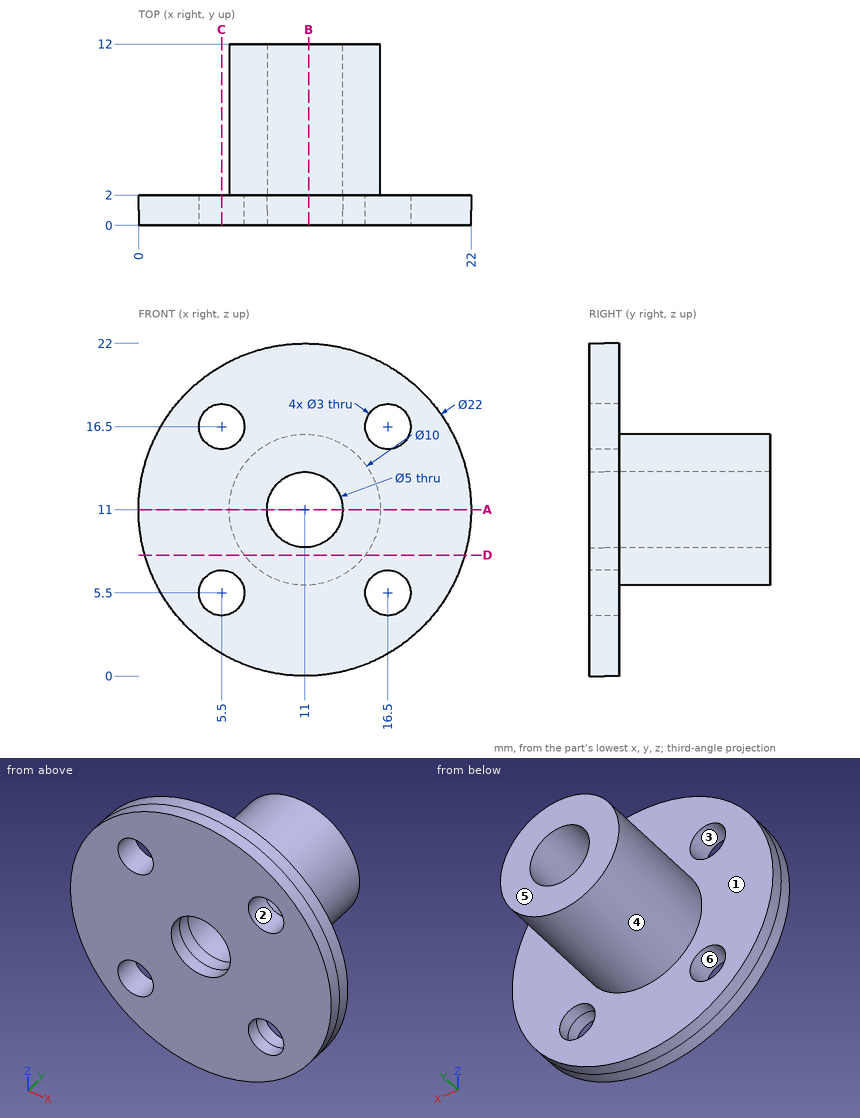
Part print with two shaded views. Sizes in mm from the minimum x, y, z corner. A direction names the side the tool comes from. Coordinates: 2 decimals unless noted, no trailing zeros. Write each loop counter-clockwise with the first axis right and the second up, starting at its lowest first coordinate (ties: lowest second). Pieces come first, ordered by that corner, then holes. Notation, with made-up numbers: (38, -8.75) -> (47, -8.75) arc R12 ccw to (47, 4.25) -> close; hole circle Ø10 at (-17, 51.5). An arc over 180 degrees is marked (long way). Return JSON: item names as keys, results as strings. Group by question number.
Q1. Flat gauge pins, fed straight in: pin 1 (2.5 mm diameter, centred on x = 16.5, z = 5.5, fed in from -Y); pin 2 (3 mm diameter, centred on y = 4, z = 7.5, fed in from -X); pin 3 (1.5 mm diameter, centred on y = 8.5, z = 11.5, fed in from -X); pin 4 (3.5 mm diameter, centred on x = 5.5, z = 5.5, fed in from +Y). Where does each tip first touch, or does it go through?
Q2. Drill centre lines: line 1 (X direction, y = 5.5, z = 11); line 2 (Z direction, x = 11, y = 0.5); line 3 (Y direction, x = 13, z = 2.25). Where is each one in solid material? Low to high.
Q3. Cut at B-B, the plane x = 11.25. Give the cut face in (y, z).
Q4. Cut at A-A, the plane z = 11. Give the cut face in (x, y), then the cut area to 3 significant figures.
Q5. Which spindle directions (+Z, -Z, +X, -X, +Y, -Y) get a long thin tool onto all of the face, cutting with end or side? Do the marked faces 1 and 2. Say none if no direction does.
Q6. Cut at D-D, the plane z = 8. Give the cut face in (x, y).
Q7. Pull direction Z, two halves, no side cores. Call the marked faces 3, 4, 5 and 6: released by +Z, released by -Z, zero draft, split by the parting line, or undercut.
Q8. Cut at C-C, the plane x = 5.5. Give the cut face in (y, z).
Returned:
{
 "1": {"pin 1": "passes through", "pin 2": "stops at x = 6.42", "pin 3": "stops at x = 6", "pin 4": "stops at y = 2"},
 "2": {"line 1": "x = 6 to 8.5, 13.5 to 16", "line 2": "z = 0 to 8.5, 13.5 to 22", "line 3": "y = 0 to 2"},
 "3": {"outline": "(0, 0) -> (2, 0) -> (2, 6.01) -> (12, 6.01) -> (12, 8.51) -> (0, 8.51) -> close; (0, 13.49) -> (12, 13.49) -> (12, 15.99) -> (2, 15.99) -> (2, 22) -> (0, 22) -> close"},
 "4": {"outline": "(0, 0) -> (8.5, 0) -> (8.5, 12) -> (6, 12) -> (6, 2) -> (0, 2) -> close; (13.5, 0) -> (22, 0) -> (22, 2) -> (16, 2) -> (16, 12) -> (13.5, 12) -> close", "area": "84.0 mm2"},
 "5": {"face 1": "+Y", "face 2": "+Y, -Y"},
 "6": {"outline": "(0.42, 0) -> (21.58, 0) -> (21.58, 2) -> (15, 2) -> (15, 12) -> (7, 12) -> (7, 2) -> (0.42, 2) -> close"},
 "7": {"face 3": "undercut", "face 4": "split by the parting line", "face 5": "zero draft", "face 6": "undercut"},
 "8": {"outline": "(0, 1.47) -> (2, 1.47) -> (2, 4) -> (0, 4) -> close; (0, 7) -> (2, 7) -> (2, 15) -> (0, 15) -> close; (0, 18) -> (2, 18) -> (2, 20.53) -> (0, 20.53) -> close"}
}
